from build123d import *

# Parameters (mm, degrees)
EXTRUDE_1_DEPTH      = 5
SKETCH_3_W           = 4
SKETCH_3_H           = 42
EXTRUDE_2_DEPTH      = 42
SKETCH_4_R           = 1.5
CUT_EXTRUDE_1_DEPTH  = 42.5
SKETCH_5_R           = 12.5
CUT_EXTRUDE_2_DEPTH  = 42.5
SKETCH_6_R           = 1.5
CUT_EXTRUDE_3_DEPTH  = 42.5
SKETCH_7_W           = 20
SKETCH_7_H           = 5
EXTRUDE_3_DEPTH      = 5
EXTRUDE_5_DEPTH      = 42
SKETCH_11_W          = 20
SKETCH_11_H          = 5
EXTRUDE_6_DEPTH      = 18
SKETCH_12_W          = 4
SKETCH_12_H          = 20
EXTRUDE_7_DEPTH      = 42
CUT_EXTRUDE_4_REACH  = 106.221
SKETCH_13_R          = 1.6
CUT_EXTRUDE_START    = -22
SKETCH_15_W          = 10
SKETCH_15_H          = 27
CUT_EXTRUDE_5_DEPTH  = 22
SKETCH_16_W          = 5
SKETCH_16_H          = 5
CUT_EXTRUDE_6_DEPTH  = 42
EXTRUDE_START        = -22
SKETCH_17_W          = 10
SKETCH_17_H          = 5
EXTRUDE_8_DEPTH      = 22
CUT_EXTRUDE_7_DEPTH  = 5
FILLET_1_R           = 4
SKETCH_20_W          = 14
SKETCH_20_H          = 5
CUT_EXTRUDE_8_DEPTH  = 5
FILLET_3_R           = 3
SKETCH_21_R          = 2.9
CUT_EXTRUDE_9_DEPTH  = 3
EXTRUDE_9_DEPTH      = 4
SKETCH_24_R          = 1.5
CUT_EXTRUDE_10_DEPTH = 4
SKETCH_26_R          = 2.9
CUT_EXTRUDE_15_DEPTH = 4
CHAMFER_1_SIZE       = 7
EXTRUDE_10_REACH     = 103.064
SKETCH_28_W          = 5
SKETCH_28_H          = 10


# Some blends are built 0.0001 mm under size
with BuildPart() as part:
    # 草图1 → 凸台-拉伸1 (new body)
    with BuildSketch(Plane(origin=(0, 0, 0), x_dir=(1, 0, 0), z_dir=(0, 1, 0))):
        Polygon((10, 0), (50, 0), (50, -20), (60, -20), (60, 0), (60, 42), (0, 42), (0, 0), (0, -20), (10, -20), align=None)
    extrude(amount=EXTRUDE_1_DEPTH)

    # 草图3 → 凸台-拉伸2 (add)
    with BuildSketch(Plane(origin=(0, 5, 0), x_dir=(1, 0, 0), z_dir=(0, 1, 0))):
        with Locations((58, 21)):
            Rectangle(SKETCH_3_W, SKETCH_3_H)
    extrude(amount=EXTRUDE_2_DEPTH)

    # 草图4 → 切除-拉伸1 (cut)
    with BuildSketch(Plane.ZY.offset(-56)):
        with Locations((-36.5, 41.5)):
            Circle(SKETCH_4_R)
        with Locations((-5.5, 41.5)):
            Circle(SKETCH_4_R)
        with Locations((-5.5, 10.5)):
            Circle(SKETCH_4_R)
        with Locations((-36.5, 10.5)):
            Circle(SKETCH_4_R)
    extrude(amount=-CUT_EXTRUDE_1_DEPTH, mode=Mode.SUBTRACT)

    # 草图5 → 切除-拉伸2 (cut)
    with BuildSketch(Plane.ZY.offset(-56)):
        with Locations((-21, 26)):
            Circle(SKETCH_5_R)
    extrude(amount=-CUT_EXTRUDE_2_DEPTH, mode=Mode.SUBTRACT)

    # 草图6 → 切除-拉伸3 (cut)
    with BuildSketch(Plane(origin=(0, 5, 0), x_dir=(1, 0, 0), z_dir=(0, 1, 0))):
        with Locations(Location((55, -10, 0), (0, 0, 270))):
            Circle(SKETCH_6_R)
        with Locations(Location((5, -10, 0), (0, 0, 270))):
            Circle(SKETCH_6_R)
    extrude(amount=-CUT_EXTRUDE_3_DEPTH, mode=Mode.SUBTRACT)

    # 草图7 → 凸台-拉伸3 (add)
    with BuildSketch(Plane(origin=(60, 0, 0), x_dir=(0, 0, -1), z_dir=(1, 0, 0))):
        with Locations((-10, 2.5)):
            Rectangle(SKETCH_7_W, SKETCH_7_H)
    extrude(amount=EXTRUDE_3_DEPTH)

    # 草图8 → 凸台-拉伸5 (add)
    with BuildSketch(Plane(origin=(0, 5, 0), x_dir=(1, 0, 0), z_dir=(0, 1, 0))):
        Polygon((65, 0), (56, 0), (56, -5), (61, -5), (61, -15), (56, -15), (56, -20), (65, -20), align=None)
    extrude(amount=EXTRUDE_5_DEPTH)

    # 草图11 → 凸台-拉伸6 (add)
    with BuildSketch(Plane(origin=(65, 0, 0), x_dir=(0, 0, -1), z_dir=(1, 0, 0))):
        with Locations((-10, 2.5)):
            Rectangle(SKETCH_11_W, SKETCH_11_H)
    extrude(amount=EXTRUDE_6_DEPTH)

    # 草图12 → 凸台-拉伸7 (add)
    with BuildSketch(Plane(origin=(0, 5, 0), x_dir=(1, 0, 0), z_dir=(0, 1, 0))):
        with Locations((81, -10)):
            Rectangle(SKETCH_12_W, SKETCH_12_H)
    extrude(amount=EXTRUDE_7_DEPTH)

    # 切除-拉伸4: up to this face of the body (flat: up to its plane)
    cut_extrude_4_end = Plane(part.part.faces().sort_by_distance((61, 26, 10))[0])
    # 草图13 → 切除-拉伸4 (cut, up to the picked face)
    with BuildSketch(Plane(origin=(83, 0, 0), x_dir=(0, 0, -1), z_dir=(1, 0, 0)), mode=Mode.PRIVATE) as cut_extrude_4_sk1:
        with Locations((-10, 37)):
            Circle(SKETCH_13_R)
    cut_extrude_4_tool1 = split(extrude(cut_extrude_4_sk1.sketch, amount=-CUT_EXTRUDE_4_REACH, mode=Mode.PRIVATE), bisect_by=cut_extrude_4_end, keep=Keep.BOTH, mode=Mode.PRIVATE)
    add(cut_extrude_4_tool1.solids().sort_by(Axis((83, 37, 10), (-1, 0, 0)))[0], mode=Mode.SUBTRACT)

    # 草图15 → 切除-拉伸5 (cut)
    with BuildSketch(Plane.ZY.offset(-61).offset(CUT_EXTRUDE_START)):
        with Locations((10, 18.5)):
            Rectangle(SKETCH_15_W, SKETCH_15_H)
    extrude(amount=CUT_EXTRUDE_5_DEPTH, mode=Mode.SUBTRACT)

    # 草图16 → 切除-拉伸6 (cut)
    with BuildSketch(Plane(origin=(0, 47, 0), x_dir=(1, 0, 0), z_dir=(0, 1, 0))):
        with Locations((58.5, -17.5)):
            Rectangle(SKETCH_16_W, SKETCH_16_H)
    extrude(amount=-CUT_EXTRUDE_6_DEPTH, mode=Mode.SUBTRACT)

    # 草图17 → 凸台-拉伸8 (add)
    with BuildSketch(Plane.ZY.offset(-61).offset(EXTRUDE_START)):
        with Locations((10, 7.5)):
            Rectangle(SKETCH_17_W, SKETCH_17_H)
    extrude(amount=EXTRUDE_8_DEPTH)

    # 草图19 → 切除-拉伸7 (cut)
    with BuildSketch(Plane(origin=(0, 10, 0), x_dir=(1, 0, 0), z_dir=(0, 1, 0))):
        Polygon((79, -15), (83, -15), (83, -5), (79, -5), (65, -5), (61, -5), (61, -15), (65, -15), align=None)
    extrude(amount=-CUT_EXTRUDE_7_DEPTH, mode=Mode.SUBTRACT)

    # 圆角1
    fillet_1_edges = [part.edges().sort_by_distance(p)[0] for p in [
        (83, 23.5, 0),
        (83, 23.5, 20),
        (81, 47, 20),
        (81, 47, 0),
        (50, 2.5, 20),
        (10, 2.5, 20),
        (0, 2.5, 20),
        (58, 47, -42),
        (63, 47, 20),
    ]]
    fillet(fillet_1_edges, radius=FILLET_1_R - 0.0001)  # a hair under: the kernel refuses the full size

    # 草图20 → 切除-拉伸8 (cut)
    with BuildSketch(Plane.XY.offset(20)):
        with Locations((72, 2.5)):
            Rectangle(SKETCH_20_W, SKETCH_20_H)
    extrude(amount=-CUT_EXTRUDE_8_DEPTH, mode=Mode.SUBTRACT)

    # 圆角3
    # the kernel refuses this fillet: 3 mm, written as the material it takes off along each edge
    with BuildSketch(Plane(origin=(79, 0, 15), x_dir=(0, 0, -1), z_dir=(-1, 0, 0)), Plane(origin=(65, 5, 15), x_dir=(0, 0, -1), z_dir=(1, 0, 0))) as fillet_3_piece_1:
        with BuildLine():
            CenterArc((FILLET_3_R, -FILLET_3_R), FILLET_3_R, 90, 90)
            Line((0, -FILLET_3_R), (0, 0))
            Line((0, 0), (FILLET_3_R, 0))
        make_face()
    extrude(amount=14, mode=Mode.SUBTRACT)

    # 草图21 → 切除-拉伸9 (cut)
    with BuildSketch(Plane(origin=(0, 5, 0), x_dir=(1, 0, 0), z_dir=(0, 1, 0))):
        with Locations(Location((5, -10, 0), (0, 0, 270))):
            Circle(SKETCH_21_R)
        with Locations(Location((55, -10, 0), (0, 0, 270))):
            Circle(SKETCH_21_R)
    extrude(amount=-CUT_EXTRUDE_9_DEPTH, mode=Mode.SUBTRACT)

    # 草图23 → 凸台-拉伸9 (add)
    with BuildSketch(Plane.XZ):
        with BuildLine():
            Line((54, 20), (65, 20))
            Line((65, 20), (65, 14.958039892))
            Line((65, 14.958039892), (79, 14.958039892))
            Line((79, 14.958039892), (79, 20))
            ThreePointArc((79, 20), (81.828427125, 18.828427125), (83, 16))
            Line((83, 16), (83, 7))
            Line((83, 7), (50, 7))
            Line((50, 7), (50, 16))
            ThreePointArc((50, 16), (51.171572875, 18.828427125), (54, 20))
        make_face()
        with BuildLine():
            Line((4, 20), (6, 20))
            ThreePointArc((6, 20), (8.828427125, 18.828427125), (10, 16))
            Line((10, 16), (10, 7))
            Line((10, 7), (0, 7))
            Line((0, 7), (0, 16))
            ThreePointArc((0, 16), (1.171572875, 18.828427125), (4, 20))
        make_face()
    extrude(amount=EXTRUDE_9_DEPTH)

    # 草图24 → 切除-拉伸10 (cut)
    with BuildSketch(Plane(origin=(0, 0, 0), x_dir=(1, 0, 0), z_dir=(0, 1, 0))):
        with Locations(Location((55, -10, 0), (0, 0, 270))):
            Circle(SKETCH_24_R)
        with Locations(Location((5, -10, 0), (0, 0, 270))):
            Circle(SKETCH_24_R)
    extrude(amount=-CUT_EXTRUDE_10_DEPTH, mode=Mode.SUBTRACT)

    # 草图26 → 切除-拉伸15 (cut)
    with BuildSketch(Plane(origin=(0, 2, 0), x_dir=(1, 0, 0), z_dir=(0, 1, 0))):
        with Locations(Location((55, -10, 0), (0, 0, 270))):
            Circle(SKETCH_26_R)
        with Locations(Location((5, -10, 0), (0, 0, 270))):
            Circle(SKETCH_26_R)
    extrude(amount=-CUT_EXTRUDE_15_DEPTH, mode=Mode.SUBTRACT)

    # 倒角1
    chamfer_1_edges = [part.edges().sort_by_distance(p)[0] for p in [
        (79, 5, 2.5),
        (65, 5, 2.5),
    ]]
    chamfer(chamfer_1_edges, length=CHAMFER_1_SIZE - 0.0001)  # a hair under: the kernel refuses the full size

    # 草图28 → 凸台-拉伸10 (add, up to next)
    with BuildSketch(Plane.ZY.offset(-79), mode=Mode.PRIVATE) as extrude_10_sk1:
        with Locations((17.5, 19)):
            Rectangle(SKETCH_28_W, SKETCH_28_H)
    extrude_10_tool1 = extrude(extrude_10_sk1.sketch, amount=EXTRUDE_10_REACH, mode=Mode.PRIVATE) - part.part
    add(extrude_10_tool1.solids().sort_by_distance((79, 19, 17.5))[0])


solid = part.part
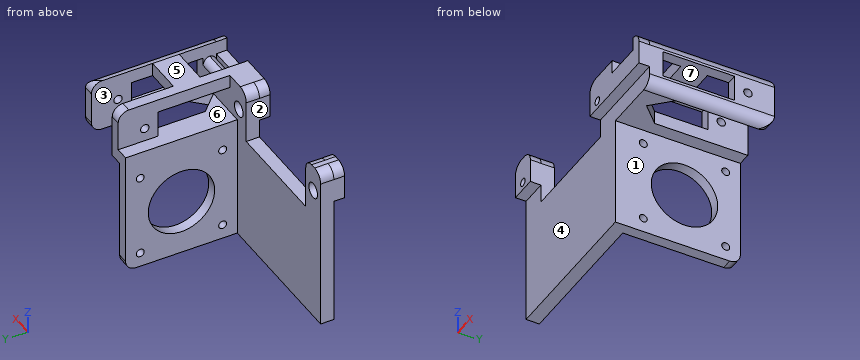
Verification items for the finished model (mm, model axes). Face numbers are marked on the shaded views. A direction names the side the tool comes from. Round coordinates to 2 decimals unless told otherwise and drop trailing zeros. Loops run counter-clockwise (first coordinate to the right, second up) from the corner with the lowest first, then second, coordinate; pieces in that order, holes last. Notation, with made-up numbers: (39.25, 18.5) - (62.25, 18.5) arc R10 ccw to (62.25, 30.5) - close; hole circle Ø8 at (-4, 11). An arc over 180 degrees is marked (long way). Use a Markdown table: item, result. Add a question column.
1. Section check C-C, the plane x = 63.5. Record the boundary of the cut face in (y, z), plus the area to 3 significant figures.
2. Section check B-B, the plane z = -21. Record the boundary of the cut face in (x, y), plus the area to 3 significant figures.
3. Access from +Z, -Z, +X, -X, +Y, -Y to the whole of each face (thin tool, end or side, straight path). Record for the marked faces 1, 2 and 3.
4. Section check D-D, the plane y = 6. Give the number of separate pieces and of enclosed holes in the cut face, plus the area to 3 significant figures.
5. Gauge pin test, flat ends, axial feed: pin 1 (4 mm diameter, centred on x = 34, y = 2.5, fed in from +Z); pin 2 (4 mm diameter, centred on y = 1, z = 16.5, fed in from +X); pin 3 (1.5 mm diameter, centred on x = 73.5, z = 18, fed in from +Y); pin 4 (6 mm diameter, centred on x = 14.5, z = -14.5, fed in from +Y). Record the tip position at first contact, or that the pin passes through.
6. Release check for a two-part mould opening along Y. For the marked faces 4, 5, 6 and 7 record: released by +Y, released by -Y, zero draft, split by the parting line, or undercut.
7. Section check A-A, the plane x = 55. Record the boundary of the cut face in (y, z), plus the area to 3 significant figures.
8. Thickness scan on probe 1 along X at (y, z) = (-3.4, 10); probe 2 along X at (y, z) = (40, 10); probe 3 along Y at (x, z) = (58.25, -5.5). Record the ranges inside material, lowest first. Write a range as [from, to].
Checks:
| question | item | result |
|---|---|---|
| 1 | outline | (-4, 7) - (0, 7) - (0, 0) - (47, 0) - (47, 16) arc R4 ccw to (43, 20) - (-4, 20) - close; hole (5, 5) - (32, 5) - (32, 15) - (5, 15) - close; hole circle Ø3.2 at (37, 10) |
| 1 | area | 711 mm^2 |
| 2 | outline | (0, 0) - (60, 0) - (60, 13.5) - (56, 13.5) - (56, 5) - (0, 5) - close; (56, 38.5) - (60, 38.5) - (60, 47) - (56, 47) - close |
| 2 | area | 368 mm^2 |
| 3 | face 1 | -Z, +X, +Y, -Y |
| 3 | face 2 | +Z, +Y, -Y |
| 3 | face 3 | -Z, +Y |
| 4 | separate pieces | 4 |
| 4 | enclosed holes | 0 |
| 4 | area | 326 mm^2 |
| 5 | pin 1 | stops at z = 0 |
| 5 | pin 2 | stops at x = 83 |
| 5 | pin 3 | stops at y = 24 |
| 5 | pin 4 | stops at y = 5 |
| 6 | face 4 | released by -Y |
| 6 | face 5 | zero draft |
| 6 | face 6 | undercut |
| 6 | face 7 | undercut |
| 7 | outline | (-4, 7) - (0, 7) - (0, -42) - (5, -42) - (5, 7.1) - (-2, 7.1) - (-2, 8.5) - (-4, 8.5) - close; (-4, 11.5) - (-2, 11.5) - (-2, 12.9) - (5, 12.9) - (5, 20) - (-4, 20) - close |
| 7 | area | 315 mm^2 |
| 8 | probe 1 | x = [0, 3.5], [6.5, 10], [50, 53.5], [56.5, 83] |
| 8 | probe 2 | x = [61, 65], [79, 83] |
| 8 | probe 3 | y = [0, 9], [12, 40], [43, 47] |
